Design review of the part built by this model. Coordinates are the model's own, in mm. A direction names the side the tool comes from. Coordinates: 2 decimals unless noted, no trailing zeros. Loops run counter-clockwise (first coordinate to the right, second up) from the corner with the lowest first, then second, coordinate; pieces in that order, holes last. Notation, with made-up numbers: M 71,37 L 81,37 A34 cw 81,67 Z; hole C 89.5,0 d11. An arc over 180 degrees is marked long. Answer as a JSON object with one key per item and string values. Group by question number.
1. To check wall thickness, follow probe 1 along Z at (x, y) = (113.5, 11.5); probe 2 along Z at (x, y) = (106, 16.5); probe 3 along Z at (x, y) = (40, 27). State the ranges of each line that lie inside material, in increasing order.
2. Machinability: for faces 5 (the flat face through (6, 18, 116.25)), 6 (the flat face through (-17, -2, 67)), 7 (the flat face through (49, 20, 84)), 8 (the flat face through (100, -2, 82.5)), which of the approach directions +Z, -Z, +X, -X, +Y, -Y give a long, thin tool a straight path to every point of the face, cutting with its end or side? Answer none if there is none.
3. Draft analysis for pull direction X (two halves, no side actions). For faces 1 (the flat face through (53, -30, 22)), 2 (the cylindrical face through (104.925, 17.535, 64.436)), 3 (the flat face through (96, 18, 112.25)), 4 (the cylindrical face through (134.993, 0.66, 22.185)), state which applies: +X half, -X half, draft (parallel to the pull), parting line (faces both ways), or undercut.
4. Consider section C-C (x = 38.2). State the section outline as (y, z) points, then the cut area to 3 significant figures.
5. Consider section B-B (z = 62.75). State the section outline as (x, y) points, then the cut area to 3 significant figures.
6. Consider section D-D (z = 106.25). State the section outline as (x, y) points.
7. Consider section A-A (y = 0). State the section outline as (x, z) points.
8. Insertion check: pin 1 (24 mm diameter, centred on x = 77, z = 77, fed in from -Y); pin 2 (4 mm diameter, centred on x = 1, y = -7.5, fed in from -Z); pin 3 (1.2 mm diameter, centred on x = 7, z = 56, fed in from +Y); pin 4 (5 mm diameter, centred on y = 16, z = 145.5, fed in from -X). Each pin has a flat end and moves straight along its axis. Give the tip position at first contact, or say it passes through.
from build123d import *

# Parameters (mm, degrees)
BOSS_EXTRU_1_DEPTH      = 170
ESQUISSE2_W             = 206.92447976
ESQUISSE2_H             = 80
ENL_V_MAT_EXTRU_1_DEPTH = 170
ESQUISSE3_W             = 140
ESQUISSE3_H             = 2.5
BOSS_EXTRU_2_DEPTH      = 80
ESQUISSE4_W             = 140
ESQUISSE4_H             = 75
BOSS_EXTRU_4_DEPTH      = 2.5
ESQUISSE5_W             = 33
ESQUISSE5_H             = 40
BOSS_EXTRU_5_DEPTH      = 34
ESQUISSE6_R             = 7
ESQUISSE6_R_2           = 2
ENL_V_MAT_EXTRU_2_DEPTH = 5


with BuildPart() as part:
    # Esquisse1 → Boss.-Extru.1 (new body)
    with BuildSketch(Plane.XY):
        with BuildLine():
            Line((0, 30), (105, 30))
            ThreePointArc((105, 30), (135, 0), (105, -30))
            Line((105, -30), (0, -30))
            ThreePointArc((0, -30), (-30, 0), (0, 30))
        make_face()
    extrude(amount=BOSS_EXTRU_1_DEPTH)

    # Esquisse2 → Enl_v. mat.-Extru.1 (cut)
    with BuildSketch(Plane(origin=(0, 30, 0), x_dir=(1, 0, 0), z_dir=(0, 1, 0))):
        with Locations((42.57058543, -85)):
            Rectangle(ESQUISSE2_W, ESQUISSE2_H)
    extrude(amount=-ENL_V_MAT_EXTRU_1_DEPTH, mode=Mode.SUBTRACT)


with BuildPart() as enl_v_mat_extru_1_piece_1:
    # of the separate pieces the step leaves, piece 1, a body of its own (enl_v_mat_extru_1_pieces)
    add(part.part.solids().sort_by_distance((105, -30, 0))[0])



with BuildPart() as enl_v_mat_extru_1_piece_2:
    # of the separate pieces the step leaves, piece 2, a body of its own (enl_v_mat_extru_1_pieces)
    add(part.part.solids().sort_by_distance((0, -30, 125))[0])


with BuildPart() as enl_v_mat_extru_1_piece_1_1:
    add(enl_v_mat_extru_1_piece_1.part)

    add(enl_v_mat_extru_1_piece_2.part)  # Boss.-Extru.2 merges Enl_v. mat.-Extru.1 piece 2
    # Esquisse3 → Boss.-Extru.2 (add)
    with BuildSketch(Plane.XY.offset(45)):
        with Locations((50, 16.25)):
            Rectangle(ESQUISSE3_W, ESQUISSE3_H)
    extrude(amount=BOSS_EXTRU_2_DEPTH)

    # Esquisse4 → Boss.-Extru.4 (add)
    with BuildSketch(Plane(origin=(0, 17.5, 0), x_dir=(1, 0, 0), z_dir=(0, 1, 0))):
        with Locations((50, -85)):
            Rectangle(ESQUISSE4_W, ESQUISSE4_H)
    extrude(amount=BOSS_EXTRU_4_DEPTH)

    # Esquisse5 → Boss.-Extru.5 (add)
    with BuildSketch(Plane.XZ.offset(-15)):
        with Locations((-0.5, 67.5)):
            Rectangle(ESQUISSE5_W, ESQUISSE5_H)
        with Locations((100.5, 102.5)):
            Rectangle(ESQUISSE5_W, ESQUISSE5_H)
    extrude(amount=BOSS_EXTRU_5_DEPTH)

    # Esquisse6 → Enl_v. mat.-Extru.2 (cut)
    with BuildSketch(Plane(origin=(0, 20, 0), x_dir=(1, 0, 0), z_dir=(0, 1, 0))):
        with Locations(Location((7, -85, 0), (0, 0, 180))):
            Circle(ESQUISSE6_R)
        with Locations(Location((23.7, -85, 0), (0, 0, 180))):
            Circle(ESQUISSE6_R_2)
        with Locations(Location((38.2, -85, 0), (0, 0, 180))):
            Circle(ESQUISSE6_R_2)
        with Locations(Location((64, -114.25, 0), (0, 0, 180))):
            Circle(ESQUISSE6_R_2)
        with Locations(Location((64, -55.616071429, 0), (0, 0, 180))):
            Circle(ESQUISSE6_R_2)
        with Locations(Location((78, -62.75, 0), (0, 0, 180))):
            Circle(ESQUISSE6_R_2)
        with Locations(Location((106, -62.75, 0), (0, 0, 180))):
            Circle(ESQUISSE6_R_2)
        with Locations(Location((106, -106.25, 0), (0, 0, 180))):
            Circle(ESQUISSE6_R_2)
        with BuildLine():
            Line((-9.5, -53.75), (21.5, -53.75))
            ThreePointArc((21.5, -53.75), (22.560660172, -54.189339828), (23, -55.25))
            Line((23, -55.25), (23, -56.25))
            ThreePointArc((23, -56.25), (22.560660172, -57.310660172), (21.5, -57.75))
            Line((21.5, -57.75), (-9.5, -57.75))
            ThreePointArc((-9.5, -57.75), (-10.560660172, -57.310660172), (-11, -56.25))
            Line((-11, -56.25), (-11, -55.25))
            ThreePointArc((-11, -55.25), (-10.560660172, -54.189339828), (-9.5, -53.75))
        make_face()
        with BuildLine():
            Line((-10.5, -69.35), (25.3, -69.35))
            ThreePointArc((25.3, -69.35), (26.360660172, -69.789339828), (26.8, -70.85))
            Line((26.8, -70.85), (26.8, -71.85))
            ThreePointArc((26.8, -71.85), (26.360660172, -72.910660172), (25.3, -73.35))
            Line((25.3, -73.35), (-10.5, -73.35))
            ThreePointArc((-10.5, -73.35), (-11.560660172, -72.910660172), (-12, -71.85))
            Line((-12, -71.85), (-12, -70.85))
            ThreePointArc((-12, -70.85), (-11.560660172, -69.789339828), (-10.5, -69.35))
        make_face()
        with BuildLine():
            Line((-10.5, -96.65), (25.3, -96.65))
            ThreePointArc((25.3, -96.65), (26.360660172, -97.089339828), (26.8, -98.15))
            Line((26.8, -98.15), (26.8, -99.15))
            ThreePointArc((26.8, -99.15), (26.360660172, -100.210660172), (25.3, -100.65))
            Line((25.3, -100.65), (-10.5, -100.65))
            ThreePointArc((-10.5, -100.65), (-11.560660172, -100.210660172), (-12, -99.15))
            Line((-12, -99.15), (-12, -98.15))
            ThreePointArc((-12, -98.15), (-11.560660172, -97.089339828), (-10.5, -96.65))
        make_face()
        with BuildLine():
            Line((-9.5, -112.25), (21.5, -112.25))
            ThreePointArc((21.5, -112.25), (22.560660172, -112.689339828), (23, -113.75))
            Line((23, -113.75), (23, -114.75))
            ThreePointArc((23, -114.75), (22.560660172, -115.810660172), (21.5, -116.25))
            Line((21.5, -116.25), (-9.5, -116.25))
            ThreePointArc((-9.5, -116.25), (-10.560660172, -115.810660172), (-11, -114.75))
            Line((-11, -114.75), (-11, -113.75))
            ThreePointArc((-11, -113.75), (-10.560660172, -112.689339828), (-9.5, -112.25))
        make_face()
        with BuildLine():
            Line((111.5, -53.75), (80.5, -53.75))
            ThreePointArc((80.5, -53.75), (79.439339828, -54.189339828), (79, -55.25))
            Line((79, -55.25), (79, -56.25))
            ThreePointArc((79, -56.25), (79.439339828, -57.310660172), (80.5, -57.75))
            Line((80.5, -57.75), (111.5, -57.75))
            ThreePointArc((111.5, -57.75), (112.560660172, -57.310660172), (113, -56.25))
            Line((113, -56.25), (113, -55.25))
            ThreePointArc((113, -55.25), (112.560660172, -54.189339828), (111.5, -53.75))
        make_face()
        with BuildLine():
            Line((80.5, -116.25), (111.5, -116.25))
            ThreePointArc((111.5, -116.25), (112.560660172, -115.810660172), (113, -114.75))
            Line((113, -114.75), (113, -113.75))
            ThreePointArc((113, -113.75), (112.560660172, -112.689339828), (111.5, -112.25))
            Line((111.5, -112.25), (80.5, -112.25))
            ThreePointArc((80.5, -112.25), (79.439339828, -112.689339828), (79, -113.75))
            Line((79, -113.75), (79, -114.75))
            ThreePointArc((79, -114.75), (79.439339828, -115.810660172), (80.5, -116.25))
        make_face()
    extrude(amount=-ENL_V_MAT_EXTRU_2_DEPTH, mode=Mode.SUBTRACT)


solid = enl_v_mat_extru_1_piece_1_1.part
Findings below:
{
 "1": {"probe 1": "z = 0 to 45, 82.5 to 122.5, 125 to 170", "probe 2": "z = 0 to 53.75, 57.75 to 60.75, 64.75 to 104.25, 108.25 to 112.25, 116.25 to 170", "probe 3": "z = 0 to 45, 125 to 170"},
 "2": {"face 5": "+Y, -Y", "face 6": "-X, -Y", "face 7": "+X, -X, +Y", "face 8": "+X, -Y"},
 "3": {"face 1": "draft", "face 2": "undercut", "face 3": "undercut", "face 4": "+X half"},
 "4": {"outline": "M -30,0 L 30,0 L 30,45 L 17.5,45 L 17.5,47.5 L 20,47.5 L 20,83 L 15,83 L 15,45 L -30,45 Z; M -30,125 L 15,125 L 15,87 L 20,87 L 20,122.5 L 17.5,122.5 L 17.5,125 L 30,125 L 30,170 L -30,170 Z", "area": "5,770 mm^2"},
 "5": {"outline": "M -20,15 L -17,15 L -17,-19 L 16,-19 L 16,15 L 76,15 L 76,20 L -20,20 Z; M 80,15 L 104,15 L 104,20 L 80,20 Z; M 108,15 L 120,15 L 120,20 L 108,20 Z", "area": "1,780 mm^2"},
 "6": {"outline": "M -20,15 L 84,15 L 84,-19 L 117,-19 L 117,15 L 120,15 L 120,20 L 108,20 L 108,15 L 104,15 L 104,20 L -20,20 Z"},
 "7": {"outline": "M -30,0 L 135,0 L 135,45 L -30,45 Z; M -30,125 L 135,125 L 135,170 L -30,170 Z; M -17,47.5 L 16,47.5 L 16,87.5 L -17,87.5 Z; M 84,82.5 L 117,82.5 L 117,122.5 L 84,122.5 Z"},
 "8": {"pin 1": "stops at y = -19", "pin 2": "stops at z = 0", "pin 3": "stops at y = 15", "pin 4": "stops at x = -26.79"}
}
